Verification items for the finished model (mm, model axes). Coordinates: 2 decimals unless noted, no trailing zeros. Write each loop counter-clockwise with the first axis right and the second up, starting at its lowest first coordinate (ties: lowest second). Pieces come first, ordered by that corner, then holes. Notation, with made-up numbers: (36, 3.25) -> (40, 3.25) arc R25 ccw to (40, 35.25) -> close; hole circle Ø6 at (3, 34.5). An arc over 180 degrees is marked (long way). Write item = value, one per line. Start each with the question number.
(1) Gauge pin test, flat ends, axial feed: pin 1 Ø8 at (x, z) = (16, 37.5) entering from +Y; pin 2 Ø5 at (x, y) = (17, -23) entering from +Z; pin 3 Ø10 at (x, y) = (23, -31.5) entering from -Z. Record the tip position at first contact, or that the pin passes through.
(2) Material ranges on probe 1 along Y at (x, z) = (13.5, 0); probe 2 along Z at (x, y) = (22, 25.5); probe 3 along Y at (x, z) = (16, 20), recorded low to high. Write a range as [from, to].
(3) Mould release check, pull along Y, two halves, no side actions. Record for faces 1 (the face through (38, -23.6, 27.5)), 2 (the face through (19, -21, 28)), 3 (the face through (17.27, 15.02, -47.69)): released by +Y, released by -Y, zero draft, split by the parting line, or undercut.
(4) Section check A-A (z = 0). Record the cut outline in (x, y).
(5) Section check C-C (x = 13). Record the cut outline in (y, z), plus the area to 3 significant figures.
```python
from build123d import *

# Parameters (mm, degrees)
SKETCH_1_R      = 50
SKETCH_1_R_2    = 35
EXTRUDE_1_DEPTH = 38
CHAMFER_1_SIZE  = 1
CHAMFER_2_SIZE  = 4


with BuildPart() as part:
    # 草图1 → 凸台-拉伸1 (new body)
    with BuildSketch(Plane(origin=(0, 0, 0), x_dir=(0, 0, -1), z_dir=(1, 0, 0))):
        Circle(SKETCH_1_R)
        Circle(SKETCH_1_R_2, mode=Mode.SUBTRACT)
    extrude(amount=EXTRUDE_1_DEPTH)

    # 倒角1
    chamfer_1_edges = [part.edges().sort_by_distance(p)[0] for p in [
        (0, 0, 50),
        (0, 0, 35),
        (38, 0, 35),
    ]]
    chamfer(chamfer_1_edges, length=CHAMFER_1_SIZE)

    # 倒角2
    chamfer_2_edges = [part.edges().sort_by_distance(p)[0] for p in [
        (38, 0, 50),
    ]]
    chamfer(chamfer_2_edges, length=CHAMFER_2_SIZE)


solid = part.part
```
Response:
q1.pin_1 = 37.12
q1.pin_2 = 45.6
q1.pin_3 = -42.4
q2.probe_1 = [-50, -35], [35, 50]
q2.probe_2 = [-43.01, -23.97], [23.97, 43.01]
q2.probe_3 = [-45.83, -28.72], [28.72, 45.83]
q3.face_1 = zero draft
q3.face_2 = undercut
q3.face_3 = split by the parting line
q4.outline = (0, -49) -> (1, -50) -> (34, -50) -> (38, -46) -> (38, -36) -> (37, -35) -> (1, -35) -> (0, -36) -> close; (0, 36) -> (1, 35) -> (37, 35) -> (38, 36) -> (38, 46) -> (34, 50) -> (1, 50) -> (0, 49) -> close
q5.outline = circle Ø100 at (0, 0); hole circle Ø70 at (0, 0)
q5.area = 4,010 mm2
